```python
from build123d import *

# Parameters (mm, degrees)
PAD010002001008_DEPTH     = 5.14
SKETCH015_W               = 71.3
SKETCH015_H               = 26.9
PAD010002001007_DEPTH     = 10.6
SKETCH014_W               = 80
SKETCH014_H               = 36
SKETCH014_R               = 1.25
SKETCH014_R_2             = 0.75
PAD010002001006_DEPTH     = 1.65
FUSION006_PLACEMENT_ANGLE = 180


with BuildPart() as displayinsert:
    # Sketch016 → Pad010002001008 (new body)
    with BuildSketch(Plane(origin=(4.5, 1.1, 0), x_dir=(1, 0, 0), z_dir=(0, 0, 1))):
        Polygon((31.5, 13.45), (-31.5, 13.45), (-41.8, 6.8), (-41.8, -6.8), (-31.5, -13.45), (31.5, -13.45), (31.5, -9.1), (32.4, -9.1), (32.4, 9.1), (31.5, 9.1), align=None)
    extrude(amount=PAD010002001008_DEPTH)


with BuildPart() as displaybody:
    # Sketch015 → Pad010002001007 (new body)
    with BuildSketch(Plane(origin=(0.45, 1.1, 0), x_dir=(1, 0, 0), z_dir=(0, 0, 1))):
        Rectangle(SKETCH015_W, SKETCH015_H)
    extrude(amount=PAD010002001007_DEPTH)


with BuildPart() as display:
    # Sketch014 → Pad010002001006 (new body)
    with BuildSketch(Plane.XY):
        Rectangle(SKETCH014_W, SKETCH014_H)
        with Locations((-37.5, 15.5)):
            Circle(SKETCH014_R, mode=Mode.SUBTRACT)
        with Locations((-37.5, -15.5)):
            Circle(SKETCH014_R, mode=Mode.SUBTRACT)
        with Locations((37.5, -15.5)):
            Circle(SKETCH014_R, mode=Mode.SUBTRACT)
        with Locations((37.5, 15.5)):
            Circle(SKETCH014_R, mode=Mode.SUBTRACT)
        with Locations((-31.197892, 15.46)):
            Circle(SKETCH014_R_2, mode=Mode.SUBTRACT)
        with Locations((-28.657892, 15.46)):
            Circle(SKETCH014_R_2, mode=Mode.SUBTRACT)
        with Locations((-26.117892, 15.46)):
            Circle(SKETCH014_R_2, mode=Mode.SUBTRACT)
        with Locations((-23.577892, 15.46)):
            Circle(SKETCH014_R_2, mode=Mode.SUBTRACT)
        with Locations((-20.413733, 15.46)):
            Circle(SKETCH014_R_2, mode=Mode.SUBTRACT)
        with Locations((-17.707897, 15.46)):
            Circle(SKETCH014_R_2, mode=Mode.SUBTRACT)
        with Locations((-15.036319, 15.46)):
            Circle(SKETCH014_R_2, mode=Mode.SUBTRACT)
        with Locations((-11.713964, 15.46)):
            Circle(SKETCH014_R_2, mode=Mode.SUBTRACT)
        with Locations((-8.905379, 15.540887)):
            Circle(SKETCH014_R_2, mode=Mode.SUBTRACT)
        with Locations((-6.268049, 15.472383)):
            Circle(SKETCH014_R_2, mode=Mode.SUBTRACT)
        with Locations((-3.767722, 15.438133)):
            Circle(SKETCH014_R_2, mode=Mode.SUBTRACT)
        with Locations((-1.4044, 15.472383)):
            Circle(SKETCH014_R_2, mode=Mode.SUBTRACT)
        with Locations((1.198681, 15.472383)):
            Circle(SKETCH014_R_2, mode=Mode.SUBTRACT)
        with Locations((4.189797, 15.510243)):
            Circle(SKETCH014_R_2, mode=Mode.SUBTRACT)
        with Locations((6.484617, 15.407489)):
            Circle(SKETCH014_R_2, mode=Mode.SUBTRACT)
        with Locations((9.361704, 15.47599)):
            Circle(SKETCH014_R_2, mode=Mode.SUBTRACT)
    extrude(amount=PAD010002001006_DEPTH)

    # Fusion005: union DisplayBody
    add(displaybody.part)

    # Fusion006: union DisplayInsert
    add(displayinsert.part)


with BuildPart() as display_1:
    # Fusion006 placement: moved
    add(display.part.moved(Location((0, -7, 44))).rotate(Axis((0, -7, 44), (0, 0, 1)), FUSION006_PLACEMENT_ANGLE))


solid = display_1.part
```
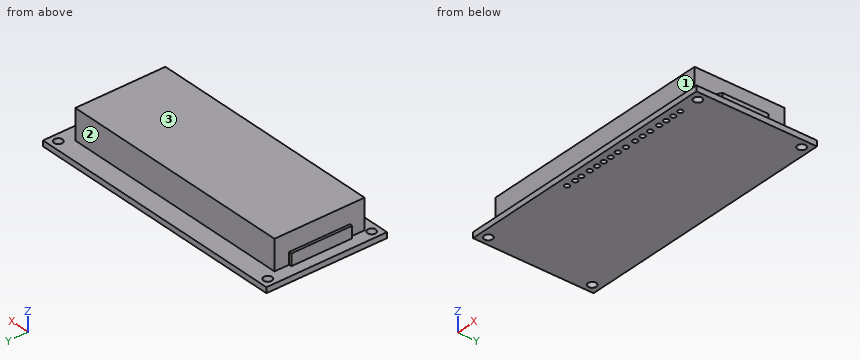
Can you work these out from the model? Positions are in its coordinate system, mm. Face numbers are marked on the shaded views. A direction names the side the tool comes from. Give positions to 0.01 mm unless a question says otherwise; leave off trailing zeros. Order: outer loops, then holes, each group sorted by start corner. A loop starts at its lowest first (then second) coordinate and runs counter-clockwise, first axis right, second up. Notation, with made-up numbers: M 16,44.25 L 72,44.25 A31 ccw 72,75.25 Z; hole C 70,-7.75 d1. An arc over 180 degrees is marked long. Write item = value, one per line. Start each with the question number.
Q1. Suppose I cut it at A-A (y = 8.5). Write out the boundary of the cut face in (x, z), plus the area to 3 significant figures.
Q2. Suppose I cut it at D-D (x = -31.5). Write out the boundary of the cut face in (y, z), plus the area to 3 significant figures.
Q3. Suppose I cut it at B-B (y = -20). Write out the boundary of the cut face in (x, z), plus the area to 3 significant figures.
Q4. For the marked faces 1, 2 and 3, which set-ups out of +Z, -Z, +X, -X, +Y, -Y let a thin tool reach every point of the face, with its end or its side?
Q5. Will these pins go through, and if not, where does the flat tip stop? pin 1 Ø2 at (x, y) = (23.58, -22.46) entering from -Z; pin 2 Ø2 at (x, z) = (2.5, 48.5) entering from -Y; pin 3 Ø3 at (x, z) = (-24, 47.5) entering from +Y; pin 4 Ø4.5 at (x, z) = (-4.5, 51.5) entering from +Y.
Q6. I need wall thicknesses on probe 1 along X at (y, z) = (-3, 54.25); probe 2 along Y at (x, z) = (2, 52); probe 3 along Y at (x, z) = (23.5, 45). Which ranges of each line are inside material? Lowest first, please. Write a range as [from, to].
Q7. Suppose I cut it at C-C (z = 47.5). Write out the boundary of the cut face in (x, y).
Check result:
q1.outline = M -40,44 L -38.75,44 L -38.75,45.65 L -40,45.65 Z; M -36.25,44 L 36.25,44 L 36.25,45.65 L -36.25,45.65 Z; M 38.75,44 L 40,44 L 40,45.65 L 38.75,45.65 Z
q1.area = 124 mm2
q2.outline = M -25,44 L 11,44 L 11,45.65 L 5.35,45.65 L 5.35,54.6 L -21.55,54.6 L -21.55,45.65 L -25,45.65 Z
q2.area = 300 mm2
q3.outline = M -40,44 L 40,44 L 40,45.65 L 35.2,45.65 L 35.2,54.6 L -36.1,54.6 L -36.1,45.65 L -40,45.65 Z
q3.area = 770 mm2
q4.face_1 = +Z, +X, -X, -Y
q4.face_2 = +Z, +X, -X, +Y
q4.face_3 = +Z, +X, -X, +Y, -Y
q5.pin_1 = 44
q5.pin_2 = -21.55
q5.pin_3 = 5.35
q5.pin_4 = 5.35
q6.probe_1 = [-36.1, 35.2]
q6.probe_2 = [-21.55, 5.35]
q6.probe_3 = [-25, -23.21], [-21.71, 11]
q7.outline = M -36.9,-17.2 L -36.1,-17.2 L -36.1,-21.55 L 35.2,-21.55 L 35.2,-16.26 L 37.3,-14.9 L 37.3,-1.3 L 35.2,0.06 L 35.2,5.35 L -36.1,5.35 L -36.1,1 L -36.9,1 Z
